Model file for the job. Use its own axes, mm. A direction names the side the tool comes from. Coordinates: 2 decimals unless noted, no trailing zeros. Loops run counter-clockwise (first coordinate to the right, second up) from the corner with the lowest first, then second, coordinate; pieces in that order, holes last. Notation, with made-up numbers: (72.25, 52.5) -> (128.25, 52.5) arc R24 ccw to (128.25, 83.5) -> close; hole circle Ø9 at (-8, 33.5). An arc over 180 degrees is marked (long way). Use one line per item in the form item = value.
Autodesk Inventor part; units mm, degrees
ref_plane "YZ Plane" through (0, 0, 0) normal (1, 0, 0) x (0, 1, 0)
ref_plane "XZ Plane" through (0, 0, 0) normal (0, 1, 0) x (-1, 0, 0)
ref_plane "XY Plane" through (0, 0, 0) normal (0, 0, 1) x (1, 0, 0)
sketch "Sketch1" plane through (0, 0, 0) normal (0, 0, 1) x (1, 0, 0)
  line L0 (-22.5, 30) -> (22.5, 30)
  line L1 (22.5, 30) -> (22.5, -30)
  line L2 (22.5, -30) -> (-22.5, -30)
  line L3 (-22.5, -30) -> (-22.5, 30)
  line L4 (-22.5, 30) -> (22.5, -30) construction
  line L5 (22.5, 30) -> (-22.5, -30) construction
  line L6 (-15, 33) -> (15, 33)
  line L7 (15, 33) -> (15, 30)
  line L8 (15, 30) -> (-15, 30)
  line L9 (-15, 30) -> (-15, 33)
  line L10 (-15, 33) -> (15, 30) construction
  line L11 (15, 33) -> (-15, 30) construction
  line L12 (-15, -30) -> (15, -30)
  line L13 (15, -30) -> (15, -33)
  line L14 (15, -33) -> (-15, -33)
  line L15 (-15, -33) -> (-15, -30)
  line L16 (-15, -30) -> (15, -33) construction
  line L17 (15, -30) -> (-15, -33) construction
  point P0 (0, 0)
  point P1 (0, 31.5)
  point P2 (0, -31.5)
  dimension "d0" = 45
  dimension "d1" = 60
  dimension "d2" = 3
  dimension "d3" = 30
extrude "Extrusion1" add sketch "Sketch1" along normal blind 3
properties part number "UNION_SOPORTE" material "MDF Medium Density Fiberboard"
Q1. Wall check: line 1 along Y through (x, z) = (-19, 1.65). Give the ranges that are in metal, low to high.
Result:
line_1 = -30 to 30
Q2. Pin check, flat tips, straight feed: pin 1 Ø1 at (x, z) = (-16, 1.5) entering from +Y; pin 2 Ø0.9 at (y, z) = (31, 1.5) entering from -X; pin 3 Ø0.9 at (x, z) = (-20, 1) entering from -Y; pin 4 Ø10 at (x, y) = (4, -18) entering from -Z. Stop position of each tip, or through.
Result:
pin_1 = 30
pin_2 = -15
pin_3 = -30
pin_4 = 0
Q3. Band-saw the part on A-A, the plane z = 1.7. Write the cut outline in (x, y), and give its area (3 significant figures).
Result:
outline = (-22.5, -30) -> (-15, -30) -> (-15, -33) -> (15, -33) -> (15, -30) -> (22.5, -30) -> (22.5, 30) -> (15, 30) -> (15, 33) -> (-15, 33) -> (-15, 30) -> (-22.5, 30) -> close
area = 2,880 mm2
Q4. Band-saw the part on B-B, the plane x = -17. Write the cut outline in (y, z), and give its area (3 significant figures).
Result:
outline = (-30, 0) -> (30, 0) -> (30, 3) -> (-30, 3) -> close
area = 180 mm2
Q5. Which spindle directions (+Z, -Z, +X, -X, +Y, -Y) get a long thin tool onto all of the face, cutting with end or side? Do faces 1 (the face through (15, -31, 1)), 2 (the face through (-19, -30, 1)), 3 (the face through (-19, 30, 1)), 4 (the face through (15, 32, 1)). Say none if no direction does.
Result:
face_1 = +Z, -Z, +X, -Y
face_2 = +Z, -Z, -X, -Y
face_3 = +Z, -Z, -X, +Y
face_4 = +Z, -Z, +X, +Y
